Here's how the part is built. I have some questions about the finished solid (model axes, mm). A direction names the side the tool comes from. Round coordinates to 2 decimals unless told otherwise and drop trailing zeros. Loops run counter-clockwise (first coordinate to the right, second up) from the corner with the lowest first, then second, coordinate; pieces in that order, holes last. Notation, with made-up numbers: M 23.5,86 L 49.5,86 A11 ccw 49.5,92 Z; hole C -27,59 d7. An arc over 180 degrees is marked long. Answer as a JSON object with one key per item and string values.
from build123d import *

# Parameters (mm, degrees)
BOSS_EXTRUDE1_DEPTH = 38.1
SKETCH2_R           = 3.3782
CUT_EXTRUDE1_DEPTH  = 18.0815


with BuildPart() as part:
    # Sketch1 → Boss-Extrude1 (new body)
    with BuildSketch(Plane(origin=(0, 0, 0), x_dir=(1, 0, 0), z_dir=(0, 1, 0))):
        with BuildLine():
            Line((-0.008466667, -16.890997878), (-19.693466667, -16.890997878))
            Line((-19.693466667, -16.890997878), (-19.693466667, 78.359002122))
            Line((-19.693466667, 78.359002122), (-26.043466667, 78.359002122))
            Line((-26.043466667, 78.359002122), (-26.043466667, -23.240997878))
            Line((-26.043466667, -23.240997878), (0, -23.240997878))
            ThreePointArc((0, -23.240997878), (23.238651666, -0.33022889), (0.660391106, 23.231613503))
            Line((0.660391106, 23.231613503), (-8.961966667, 23.231613503))
            Line((-8.961966667, 23.231613503), (-8.961966667, 78.359002122))
            Line((-8.961966667, 78.359002122), (-15.311966667, 78.359002122))
            Line((-15.311966667, 78.359002122), (-15.311966667, 16.881613503))
            Line((-15.311966667, 16.881613503), (0.563033333, 16.881613503))
            ThreePointArc((0.563033333, 16.881613503), (16.888582117, -0.285788522), (-0.008466667, -16.890997878))
        make_face()
    extrude(amount=BOSS_EXTRUDE1_DEPTH)

    # Sketch2 → Cut-Extrude1 (cut, through all)
    with BuildSketch(Plane(origin=(-8.961966667, 0, 0), x_dir=(0, 0, -1), z_dir=(1, 0, 0))):
        with Locations((72.009002122, 31.75)):
            Circle(SKETCH2_R)
        with Locations((72.389957145, 6.352856986)):
            Circle(SKETCH2_R)
    extrude(amount=-CUT_EXTRUDE1_DEPTH, mode=Mode.SUBTRACT)


solid = part.part
Item 1: Please list where these lines run through material, in increasing order: probe 1 along Y at (x, z) = (-15, -72); probe 2 along Z at (x, y) = (-20, 32); probe 3 along X at (y, z) = (20, -24.5). Write a range as from..to.
Resolved:
{"probe 1": "0..3, 9.71..28.37, 35.13..38.1", "probe 2": "-78.36..-75.38, -68.64..23.24", "probe 3": "-26.04..-19.69, -15.31..-8.96"}
Item 2: If we mould it in two halves opening along Z, with no side actions, what happens to faces 1 (the face through (-23, 19, -78.359)), 2 (the face through (23.226, 18.783, 0.837)), 3 (the face through (-12.09, 5.06, -75.51))? For each: pulls with the +Z half, pulls with the -Z half, needs draft (parallel to the pull), parting line crosses it, or undercut.
Resolved:
{"face 1": "pulls with the -Z half", "face 2": "parting line crosses it", "face 3": "undercut"}
Item 3: I want a section at A-A, the plane z = -26. Please give me the cut outline in (x, y).
Resolved:
{"outline": "M -26.04,0 L -19.69,0 L -19.69,38.1 L -26.04,38.1 Z; M -15.31,0 L -8.96,0 L -8.96,38.1 L -15.31,38.1 Z"}
Item 4: I'm going to push flat-ended pins straight in: pin 1 Ø6 at (x, y) = (10, 24.5) entering from -Z; pin 2 Ø8 at (x, y) = (14, 34) entering from +Z; pin 3 Ø6 at (x, y) = (16, 24.5) entering from -Z; pin 4 Ø5.5 at (y, z) = (6.35, -72.39) entering from +X. Where does each tip first touch, or does it pass through?
Resolved:
{"pin 1": "z = -22.16", "pin 2": "z = 20.98", "pin 3": "z = -19.27", "pin 4": "through"}
Item 5: I want a section at B-B, the plane x = -3. Please give me the cut outline in (y, z).
Resolved:
{"outline": "M 0,-23.23 L 38.1,-23.23 L 38.1,-16.88 L 0,-16.88 Z; M 0,16.89 L 38.1,16.89 L 38.1,23.24 L 0,23.24 Z"}
Item 6: I want a section at C-C, the plane y = 31.75. Please give me the cut outline in (x, z), then the cut area to 3 significant figures.
Resolved:
{"outline": "M -26.04,-78.36 L -19.69,-78.36 L -19.69,-75.39 L -26.04,-75.39 Z; M -26.04,-68.63 L -19.69,-68.63 L -19.69,16.89 L -0.01,16.89 A16.89 cw 0.56,-16.88 L -15.31,-16.88 L -15.31,-68.63 L -8.96,-68.63 L -8.96,-23.23 L 0.66,-23.23 A23.24 ccw 0,23.24 L -26.04,23.24 Z; M -15.31,-78.36 L -8.96,-78.36 L -8.96,-75.39 L -15.31,-75.39 Z", "area": "1,530 mm²"}
Item 7: On a 3-axis mill with a long thin cutter (end or side, diameter ignored), from which of +Z, -Z, +X, -X, +Y, -Y can I reach the whole of each face in a straight line? I mean faces 4 (the face through (16.89, 18.78, -0.08)), 5 (the face through (-15.312, 19, -48)), 6 (the face through (-4, 19, -23.232)). Say none if no direction works.
Resolved:
{"face 4": "+Y, -Y", "face 5": "-Z, +Y, -Y", "face 6": "-Z, +X, +Y, -Y"}
Item 8: I want a section at D-D, the plane y = 22.5. Please give me the cut outline in (x, z).
Resolved:
{"outline": "M -26.04,-78.36 L -19.69,-78.36 L -19.69,16.89 L -0.01,16.89 A16.89 cw 0.56,-16.88 L -15.31,-16.88 L -15.31,-78.36 L -8.96,-78.36 L -8.96,-23.23 L 0.66,-23.23 A23.24 ccw 0,23.24 L -26.04,23.24 Z"}
